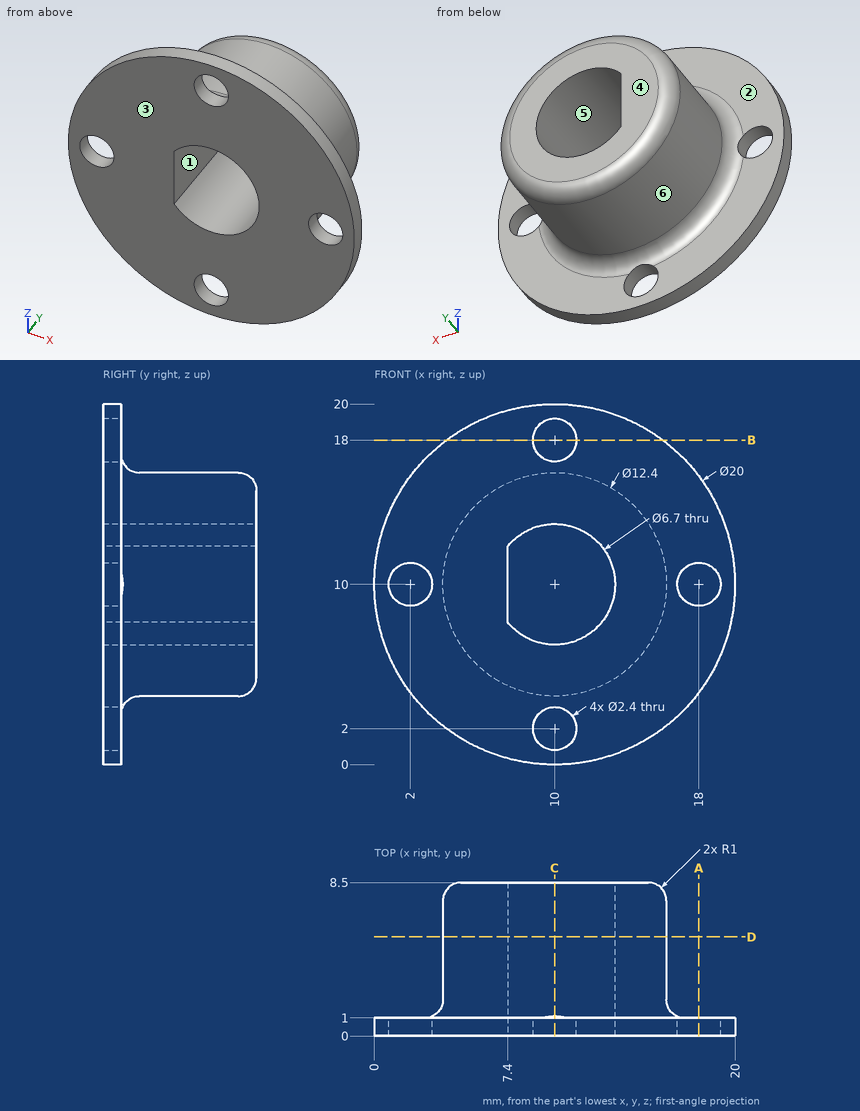
Study the drawing (mm; zero at the part's minimum x, y, z) and answer. A direction names the side the tool comes from. Coordinates: 2 decimals unless noted, no trailing zeros. Write each loop counter-clockwise with the first axis right and the second up, starting at its lowest first coordinate (ties: lowest second). Pieces come first, ordered by that corner, then holes.
Q1. Determine the mould class of the marked faces 4, 5 and 6 for opening direction Z: released by +Z, released by -Z, zero draft, split by the parting line, or undercut.
Q2. Each of these flat-tipped pins is pushed along its axis until it touches: pin 1 Ø1.5 at (x, y) = (6.5, 1.5) entering from +Z; pin 2 Ø2 at (y, z) = (2.5, 8.5) entering from -X; pin 3 Ø8.5 at (x, z) = (10, 10) entering from -Y; pin 4 Ø4 at (x, z) = (2, 10) entering from +Y. Where does it stop, or does it pass through?
Q3. A cutting plane is placed at D-D, the plane y = 5.5. Give the vertices of the cut face in (x, z), then the cut area to 3 significant figures.
Q4. A cutting plane is placed at A-A, the plane x = 18. Give the vertices of the cut face in (y, z), then the cut area to 3 significant figures.
Q5. A cutting plane is placed at C-C, the plane x = 10. Give the vertices of the cut face in (y, z), then the cut area to 3 significant figures.
Q6. A cutting plane is placed at B-B, the plane z = 18. Give the vertices of the cut face in (x, y), then the cut area to 3 significant figures.
Q7. Find the intervals of material crossed by line 1 (Y direction, x = 17.5, z = 7); line 2 (Z direction, x = 11, y = 4.25); line 3 (X direction, y = 3.25, z = 9.5), in increasing order.
Q8. Which of the six approach directions +Z, -Z, +X, -X, +Y, -Y give full straight-line access (tool end or side, diameter ignored) to the marked faces 1, 2 and 3?
Findings below:
1. face 4: zero draft
1. face 5: undercut
1. face 6: split by the parting line
2. pin 1: stops at z = 19.56
2. pin 2: stops at x = 3.81
2. pin 3: stops at y = 0
2. pin 4: stops at y = 8.1
3. outline: circle Ø12.4 at (10, 10); hole (7.4, 7.89) arc R3.35 ccw (long way) to (7.4, 12.11) - close
3. area: 87.7 mm2
4. outline: (0, 4) - (1, 4) - (1, 8.8) - (0, 8.8) - close; (0, 11.2) - (1, 11.2) - (1, 16) - (0, 16) - close
4. area: 9.60 mm2
5. outline: (0, 0) - (1, 0) - (1, 0.8) - (0, 0.8) - close; (0, 3.2) - (1.08, 3.2) arc R1 cw to (2, 3.8) - (7.5, 3.8) arc R1 ccw to (8.5, 4.8) - (8.5, 6.65) - (0, 6.65) - close; (0, 13.35) - (8.5, 13.35) - (8.5, 15.2) arc R1 ccw to (7.5, 16.2) - (2, 16.2) arc R1 cw to (1.08, 16.8) - (0, 16.8) - close; (0, 19.2) - (1, 19.2) - (1, 20) - (0, 20) - close
5. area: 51.2 mm2
6. outline: (4, 0) - (8.8, 0) - (8.8, 1) - (4, 1) - close; (11.2, 0) - (16, 0) - (16, 1) - (11.2, 1) - close
6. area: 9.60 mm2
7. line 1: y = 0 to 1
7. line 2: z = 3.88 to 6.8, 13.2 to 16.12
7. line 3: x = 3.82 to 7.4, 13.31 to 16.18
8. face 1: +Y, -Y
8. face 2: +Y
8. face 3: +Z, -Z, +X, -X, -Y
